Verification items for this drawing (mm, ordinates from the low corner). Round coordinates to 2 decimals unless told otherwise and drop trailing zeros. Loops run counter-clockwise (first coordinate to the right, second up) from the corner with the lowest first, then second, coordinate; pieces in that order, holes last. Notation, with made-up numbers: (23, -35.75) - (37, -35.75) arc R38 cw to (37, 2.25) - close; hole circle Ø5 at (-17, -33). An arc over 180 degrees is marked (long way). Put each result on its own line as item: value.
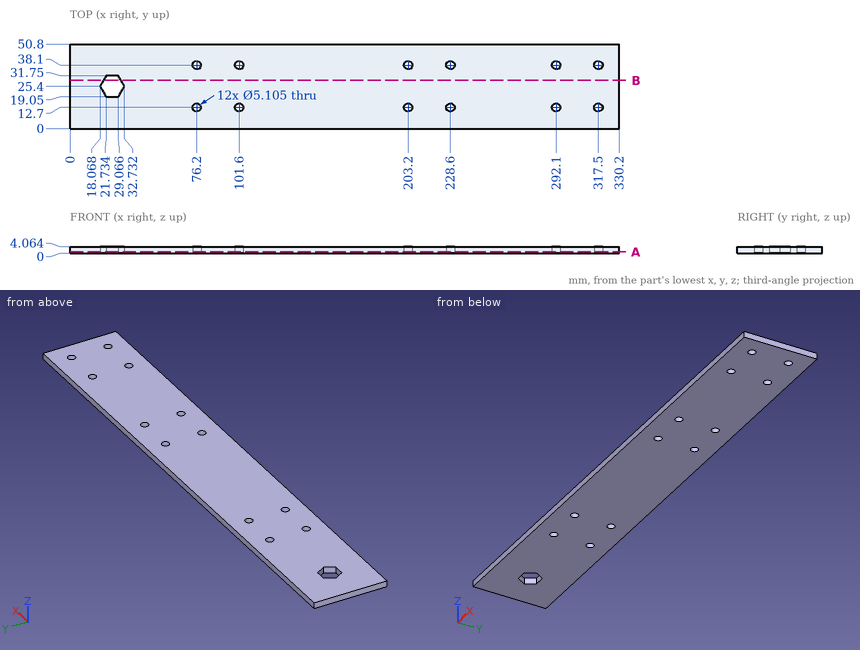
Item 1: Section check A-A on z = 0.8. Count the separate pieces of the cut face and the enclosed holes in it, then the cut area to 3 significant figures.
Filled sheet:
separate pieces: 1
enclosed holes: 13
area: 16,400 mm²
Item 2: Thickness scan on line 1 (Y direction, x = 228.6, z = 1.8); line 2 (X direction, y = 27, z = 2.65); line 3 (Y direction, x = 30.5, z = 2.2) (1 decimal). Record the ranges inside material, lowest first. Write a range as from..to.
Filled sheet:
line 1: 0..10.15, 15.25..35.55, 40.65..50.8
line 2: 0..18.99, 31.81..330.2
line 3: 0..21.5, 29.3..50.8
Item 3: Section check B-B on y = 29. Enter the section's corners in (x, z), then the cut area to 3 significant figures.
Filled sheet:
outline: (0, 0) - (20.15, 0) - (20.15, 4.06) - (0, 4.06) - close; (30.65, 0) - (330.2, 0) - (330.2, 4.06) - (30.65, 4.06) - close
area: 1,300 mm²
Item 4: Go/stop test with a flat-tipped pin: pin 1 (1.2 mm diameter, centred on x = 26.5, z = 1.5, fed in from -Y). Record where the tip stops, or that it passes through.
Filled sheet:
pin 1: y = 0
